Answer from the drawing. Dimensions are ordinates in mm from the lowest x, y and z of the part. A direction names the side the tool comes from. Give positions to 0.01 mm unless a question says otherwise; leave off trailing zeros. Loops run counter-clockwise (first coordinate to the right, second up) from the corner with the lowest first, then second, coordinate; pieces in that order, holes last. Notation, with made-up numbers: (36, -26.75) - (89, -26.75) arc R22 ccw to (89, -1.75) - close; hole circle Ø7 at (12.25, 24.5). An arc over 180 degrees is marked (long way). Put each result on its own line as item: value. Start each with the question number.
1. For a pull along X with two mould halves and no side action, classify the marked faces 4, 5 and 6 as released by +X, released by -X, zero draft, split by the parting line, or undercut.
2. A cutting plane is placed at B-B, the plane y = 18.5. Count the separate pieces of the cut face and the enclosed holes in it, plus the area to 3 significant figures.
3. Consider L1, parallel to X at y = 2.5, z = 55 (1 decimal); L2, parallel to Y at x = 52, z = 44.5; L3, parallel to Z at x = 23, y = 9 (1 decimal). Determine where each line is inside the solid, lowest interval first. Write a range as from..to.
4. For the marked faces 1, 2 and 3, determine the directions among +Z, -Z, +X, -X, +Y, -Y from which every point of the face is accessible in a straight line to the end or side of a thin tool.
5. Given pin 1 Ø3 at (y, z) = (20.5, 65.5) entering from -X; pin 2 Ø1 at (y, z) = (18, 21) entering from +X; pin 3 Ø3 at (y, z) = (17.5, 36) entering from -X, each flat-ended and moving along its own axis, determine where each tip first touches the part or whether it passes through.
6. A cutting plane is placed at D-D, the plane x = 51. Determine the outline of the cut face in (y, z), plus the area to 3 significant figures.
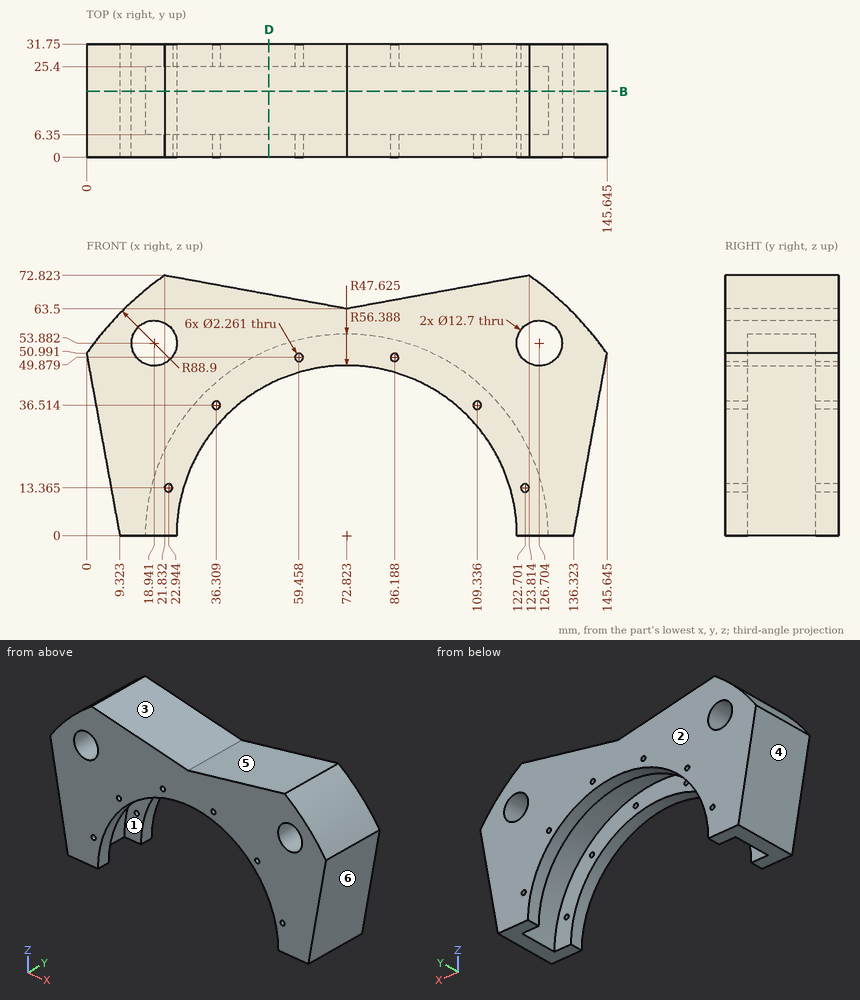
Return value:
1. face 4: released by -X
1. face 5: undercut
1. face 6: released by +X
2. separate pieces: 1
2. enclosed holes: 2
2. area: 3,990 mm2
3. L1: x = 3..12.7, 25.2..120.5, 133..142.7
3. L2: y = 0..6.35, 25.4..31.75
3. L3: z = 26.4..49, 58.8..72.6
4. face 1: -Z
4. face 2: +Z, -Z, +X, -X, +Y
4. face 3: +Z, +Y, -Y
5. pin 1: stops at x = 11.12
5. pin 2: stops at x = 140.25
5. pin 3: stops at x = 2.47
6. outline: (0, 42.33) - (6.35, 42.33) - (6.35, 51.99) - (25.4, 51.99) - (25.4, 42.33) - (31.75, 42.33) - (31.75, 67.49) - (0, 67.49) - close
6. area: 615 mm2
